Check sheet for the modelled part. Datum: model origin and axes. Units: mm. Face numbers are marked on the shaded views. A direction names the side the tool comes from. Round coordinates to 2 decimals unless told otherwise and drop trailing zeros. Loops run counter-clockwise (first coordinate to the right, second up) from the corner with the lowest first, then second, coordinate; pieces in that order, holes last. Notation, with made-up numbers: (52.5, -12) -> (101.5, -12) arc R21 ccw to (101.5, 17) -> close; hole circle Ø11 at (45, 36.25). An arc over 180 degrees is marked (long way). Return JSON: item names as keys, results as strings.
from build123d import *

# Parameters (mm, degrees)
EXTRUDE_1_DEPTH     = 11.5
SKETCH_2_R          = 1.65
CUT_EXTRUDE_1_DEPTH = 46.5
SKETCH_4_R          = 6.5
CUT_EXTRUDE_2_DEPTH = 5
SKETCH_5_W          = 7
SKETCH_5_H          = 2
CUT_EXTRUDE_3_DEPTH = 10
FILLET_1_R          = 1
CUT_EXTRUDE_4_DEPTH = 25
FILLET_2_R          = 1


with BuildPart() as part:
    # 草图1 → 凸台-拉伸1 (new, symmetric)
    with BuildSketch(Plane(origin=(0, 0, 0), x_dir=(1, 0, 0), z_dir=(0, 1, 0))):
        with BuildLine():
            Line((-12.5, 3.5), (12.5, 3.5))
            ThreePointArc((12.5, 3.5), (16, 0), (12.5, -3.5))
            Line((12.5, -3.5), (-12.5, -3.5))
            ThreePointArc((-12.5, -3.5), (-16, 0), (-12.5, 3.5))
        make_face()
    extrude(amount=EXTRUDE_1_DEPTH, both=True)

    # 草图2 → 切除-拉伸1 (cut, symmetric)
    with BuildSketch(Plane(origin=(0, 11.5, 0), x_dir=(1, 0, 0), z_dir=(0, 1, 0))):
        with Locations(Location((12.5, 0, 0), (0, 0, 270))):
            Circle(SKETCH_2_R)
        with Locations(Location((-12.5, 0, 0), (0, 0, 270))):
            Circle(SKETCH_2_R)
    extrude(amount=CUT_EXTRUDE_1_DEPTH, both=True, mode=Mode.SUBTRACT)

    # 草图4 → 切除-拉伸2 (cut, symmetric)
    with BuildSketch(Plane(origin=(0, 11.5, 0), x_dir=(1, 0, 0), z_dir=(0, 1, 0))):
        with Locations((-12.5, 0)):
            Circle(SKETCH_4_R)
    extrude(amount=CUT_EXTRUDE_2_DEPTH, both=True, mode=Mode.SUBTRACT)

    # 草图5 → 切除-拉伸3 (cut, symmetric)
    with BuildSketch(Plane.XY.offset(3.5)):
        with Locations((12.5, 9)):
            Rectangle(SKETCH_5_W, SKETCH_5_H)
    extrude(amount=CUT_EXTRUDE_3_DEPTH, both=True, mode=Mode.SUBTRACT)

    # 圆角1
    fillet_1_edges = [part.edges().sort_by_distance(p)[0] for p in [
        (9, 8, 0),
        (9, 10, 0),
    ]]
    fillet(fillet_1_edges, radius=FILLET_1_R - 0.0001)  # a hair under: the kernel refuses the full size

    # 草图6 → 切除-拉伸4 (cut, symmetric)
    with BuildSketch(Plane.XY.offset(3.5)):
        Polygon((-10, 3.5), (-10, -7.5), (7, -7.5), (7, 7.5), (-4.022774425, 7.5), (-4.022774425, 3.5), align=None)
    extrude(amount=CUT_EXTRUDE_4_DEPTH, both=True, mode=Mode.SUBTRACT)

    # 圆角2
    fillet_2_edges = [part.edges().sort_by_distance(p)[0] for p in [
        (-10, 3.5, 0),
        (-4.022774425, 3.5, 0),
        (-4.022774425, 7.5, 0),
        (7, 7.5, 0),
        (7, -7.5, 0),
        (-10, -7.5, 0),
    ]]
    fillet(fillet_2_edges, radius=FILLET_2_R)


solid = part.part
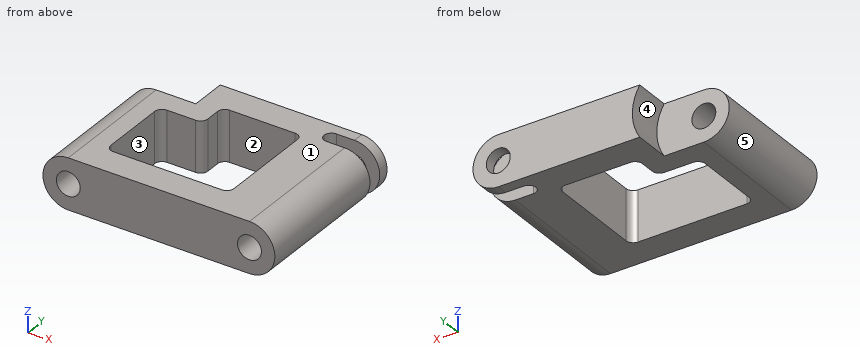
Q1. Section check B-B (y = -0.5). Record the boundary of the cut face in (x, z), then the cut area to 3 significant figures.
Results list:
{"outline": "(-12.5, -3.5) -> (-10, -3.5) -> (-10, 3.5) -> (-12.5, 3.5) arc R3.5 ccw to start; (7, -3.5) -> (12.5, -3.5) arc R3.5 ccw to (12.5, 3.5) -> (7, 3.5) -> close; hole circle Ø3.3 at (-12.5, 0); hole circle Ø3.3 at (12.5, 0)", "area": "77.4 mm^2"}
Q2. Go/stop test with flat-tipped pins: pin 1 (3.5 mm diameter, centred on x = -10.5, z = 0.5, fed in from +Y); pin 2 (2.5 mm diameter, centred on x = 12.5, z = 0, fed in from -Y). Record where each tip stops, or that it passes through.
Results list:
{"pin 1": "y = 6.5", "pin 2": "through"}
Q3. Draft check along Z on the marked faces 3, 4 and 5. Enter one of: released by +Z, released by -Z, zero draft, split by the parting line, or undercut.
Results list:
{"face 3": "zero draft", "face 4": "undercut", "face 5": "split by the parting line"}
Q4. Section check C-C (z = 0). Count the separate pieces of the cut face and the enclosed holes in it, then the cut area to 3 significant figures.
Results list:
{"separate pieces": "4", "enclosed holes": "1", "area": "313 mm^2"}
Q5. Section check A-A (x = 4). Record the boundary of the cut face in (y, z), then the cut area to 3 significant figures.
Results list:
{"outline": "(-11.5, -3.5) -> (-7.5, -3.5) -> (-7.5, 3.5) -> (-11.5, 3.5) -> close; (7.5, -3.5) -> (11.5, -3.5) -> (11.5, 3.5) -> (7.5, 3.5) -> close", "area": "56.0 mm^2"}
Q6. Material ranges on line 1 (X direction, y = 0.5, z = 0); line 2 (X direction, y = 10.95, z = 0); line 3 (Y direction, x = -3, z = 0.5), recorded low to high.
Results list:
{"line 1": "-16 to -14.15, -10.85 to -10, 7 to 10.85, 14.15 to 16", "line 2": "-6 to 10.85, 14.15 to 16", "line 3": "-11.5 to -7.5, 7.5 to 11.5"}
Q7. Tool access check on the marked faces 1 and 2. Record the directions out of +Z, -Z, +X, -X, +Y, -Y that give a thin tool (end or side, any length) a straight path to the whole face; none if there is none.
Results list:
{"face 1": "+Z, +X, -X, +Y, -Y", "face 2": "+Z, -Z"}
